```python
from build123d import *

# Parameters (mm, degrees)
SKETCH1_W           = 8
SKETCH1_H           = 4
SKETCH1_W_2         = 4
SKETCH1_H_2         = 8
BOSS_EXTRUDE1_DEPTH = 4


with BuildPart() as part:
    # Sketch1 → Boss-Extrude1 (new body)
    with BuildSketch(Plane.XY):
        Polygon((-13, 9), (-8, 4), (0, 4), (-5, 9), align=None)
        with Locations((-4, 2)):
            Rectangle(SKETCH1_W, SKETCH1_H)
        Polygon((-13, 17), (-13, 9), (-5, 9), align=None)
        with Locations((-15, 13)):
            Rectangle(SKETCH1_W_2, SKETCH1_H_2)
    extrude(amount=BOSS_EXTRUDE1_DEPTH)


solid = part.part
```
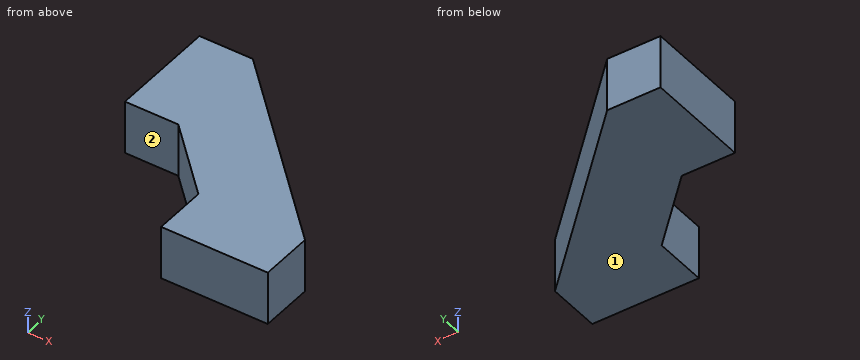
Here's how the part is built. I have some questions about the finished solid (model axes, mm). Face numbers are marked on the shaded views. A direction names the side the tool comes from. Coordinates: 2 decimals unless noted, no trailing zeros. Order: outer loops, then holes, each group sorted by start corner. A loop starts at its lowest first (then second) coordinate and runs counter-clockwise, first axis right, second up. Notation, with made-up numbers: (21.5, -5) - (60.5, -5) arc R34 cw to (60.5, 34) - close; hole circle Ø1 at (-0.75, -5). An arc over 180 degrees is marked (long way). One line per question, with ' | ' between items. Start each with the question number.
1. If we section it at A-A (z = 1.8): Write out the boundary of the cut face in (x, y), and give its area (3 significant figures).
2. If we section it at C-C (y = 10.5): Write out the boundary of the cut face in (x, z).
3. Which directions (+Z, -Z, +X, -X, +Y, -Y) give clear straight access to the entire face, cutting with the end or side of a thin tool? Please do the marked faces 1 and 2.
4. Please list where these lines run through material, in increasing order: line 1 along Y through (x, z) = (-14.75, 0.7); line 2 along X through (y, z) = (2.75, 3.35); line 3 along X through (y, z) = (14, 2.5). Write a range as [from, to].
5. If we section it at B-B (x = -2.75): Write out the boundary of the cut face in (y, z), and give its area (3 significant figures).
6. I'm going to push flat-ended pins straight in: pin 1 Ø5 at (x, y) = (-3, 8) entering from +Z; pin 2 Ø2 at (y, z) = (2, 1.5) entering from -X. Where does each tip first touch, or does it pass through?
Model answer:
1) outline: (-17, 9) - (-13, 9) - (-8, 4) - (-8, 0) - (0, 0) - (0, 4) - (-13, 17) - (-17, 17) - close | area: 136 mm²
2) outline: (-17, 0) - (-6.5, 0) - (-6.5, 4) - (-17, 4) - close
3) face 1: -Z, +X, -X, +Y, -Y | face 2: +Z, -Z, -X, -Y
4) line 1: y = [9, 17] | line 2: x = [-8, 0] | line 3: x = [-17, -10]
5) outline: (0, 0) - (6.75, 0) - (6.75, 4) - (0, 4) - close | area: 27.0 mm²
6) pin 1: stops at z = 4 | pin 2: stops at x = -8
